```python
from build123d import *

# Parameters (mm, degrees)
SKETCH_1_R      = 2
SKETCH_1_R_2    = 1.5
SKETCH_1_R_3    = 5
SKETCH_1_R_4    = 0.95
SKETCH_1_W      = 8.2
SKETCH_1_H      = 4.2
EXTRUDE_1_DEPTH = 4


with BuildPart() as part:
    # 草图1 → 凸台-拉伸1 (new body)
    with BuildSketch(Plane.XY):
        with BuildLine():
            Line((-38.15, 66.25), (-38.15, 62.25))
            Line((-38.15, 62.25), (-39.45, 62.25))
            Line((-39.45, 62.25), (-39.45, 59.65))
            Line((-39.45, 59.65), (-38.15, 59.65))
            Line((-38.15, 59.65), (-38.15, 57.05))
            Line((-38.15, 57.05), (-35.15, 57.05))
            Line((-35.15, 57.05), (-35.15, 59.65))
            Line((-35.15, 59.65), (-33.85, 59.65))
            Line((-33.85, 59.65), (-33.85, 62.25))
            Line((-33.85, 62.25), (-35.15, 62.25))
            Line((-35.15, 62.25), (-35.15, 66.25))
            Line((-35.15, 66.25), (-25.65, 66.25))
            Line((-25.65, 66.25), (-25.65, 70.25))
            Line((-25.65, 70.25), (-17.65, 70.25))
            Line((-17.65, 70.25), (-17.65, 66.25))
            Line((-17.65, 66.25), (-8.15, 66.25))
            Line((-8.15, 66.25), (-8.15, 62.25))
            Line((-8.15, 62.25), (-9.45, 62.25))
            Line((-9.45, 62.25), (-9.45, 59.65))
            Line((-9.45, 59.65), (-8.15, 59.65))
            Line((-8.15, 59.65), (-8.15, 57.05))
            Line((-8.15, 57.05), (-5.15, 57.05))
            Line((-5.15, 57.05), (-5.15, 59.65))
            Line((-5.15, 59.65), (-3.85, 59.65))
            Line((-3.85, 59.65), (-3.85, 62.25))
            Line((-3.85, 62.25), (-5.15, 62.25))
            Line((-5.15, 62.25), (-5.15, 66.25))
            Line((-5.15, 66.25), (4.35, 66.25))
            Line((4.35, 66.25), (4.35, 57.55))
            Line((4.35, 57.55), (53.51460577, -41.768082641))
            ThreePointArc((53.51460577, -41.768082641), (38.475737517, -73.658373169), (10.85, -51.75))
            Line((10.85, -51.75), (-95.15, 57.55))
            Line((-95.15, 57.55), (-95.15, 66.25))
            Line((-95.15, 66.25), (-85.65, 66.25))
            Line((-85.65, 66.25), (-85.65, 70.25))
            Line((-85.65, 70.25), (-77.65, 70.25))
            Line((-77.65, 70.25), (-77.65, 66.25))
            Line((-77.65, 66.25), (-68.15, 66.25))
            Line((-68.15, 66.25), (-68.15, 62.25))
            Line((-68.15, 62.25), (-69.45, 62.25))
            Line((-69.45, 62.25), (-69.45, 59.65))
            Line((-69.45, 59.65), (-68.15, 59.65))
            Line((-68.15, 59.65), (-68.15, 57.05))
            Line((-68.15, 57.05), (-65.15, 57.05))
            Line((-65.15, 57.05), (-65.15, 59.65))
            Line((-65.15, 59.65), (-63.85, 59.65))
            Line((-63.85, 59.65), (-63.85, 62.25))
            Line((-63.85, 62.25), (-65.15, 62.25))
            Line((-65.15, 62.25), (-65.15, 66.25))
            Line((-65.15, 66.25), (-55.65, 66.25))
            Line((-55.65, 66.25), (-55.65, 70.25))
            Line((-55.65, 70.25), (-47.65, 70.25))
            Line((-47.65, 70.25), (-47.65, 66.25))
            Line((-47.65, 66.25), (-38.15, 66.25))
        make_face()
        with Locations((-20.262745434, 32.422010331)):
            Circle(SKETCH_1_R, mode=Mode.SUBTRACT)
        with Locations((6.598407643, -9.75)):
            Circle(SKETCH_1_R_2, mode=Mode.SUBTRACT)
        with Locations((33.35, -51.75)):
            Circle(SKETCH_1_R_3, mode=Mode.SUBTRACT)
        with Locations((33.35, -45.75)):
            Circle(SKETCH_1_R_4, mode=Mode.SUBTRACT)
        with Locations((33.35, -57.75)):
            Circle(SKETCH_1_R_4, mode=Mode.SUBTRACT)
        with Locations((-8.401592357, -9.75)):
            Rectangle(SKETCH_1_W, SKETCH_1_H, mode=Mode.SUBTRACT)
    extrude(amount=EXTRUDE_1_DEPTH)


solid = part.part
```
For this review, take the finished solid that the model builds, in its own axes (mm). A direction names the side the tool comes from. Round coordinates to 2 decimals unless told otherwise and drop trailing zeros. Write each loop counter-clockwise with the first axis right and the second up, starting at its lowest first coordinate (ties: lowest second). Pieces come first, ordered by that corner, then holes.
1) Take a section at C-C on x = -61. Give the boundary of the cut face in (y, z).
Answer below:
outline: (22.34, 0) - (66.25, 0) - (66.25, 4) - (22.34, 4) - close
2) For line 1 along X through (y, z) = (61, 1.45); line 2 along X through (y, z) = (-10.5, 1.4); line 3 along X through (y, z) = (33.5, 0.55), list the stretches that pass through material, from the lowest coordinate up.
Answer below:
line 1: x = -95.15 to -69.45, -63.85 to -39.45, -33.85 to -9.45, -3.85 to 4.35
line 2: x = -29.15 to -12.5, -4.3 to 5.3, 7.9 to 38.04
line 3: x = -71.83 to -21.95, -18.58 to 16.26
3) Mouldability with a two-part tool opening along Y and no side actions: class faces 4 (the face through (0, 66.25, 2)), 5 (the face through (-4.302, -10, 2)), 6 (the face through (4.35, 62, 2)), 7 (the face through (-18.415, 31.656, 1.972)) as +Y half, -Y half, draft (parallel to the pull), parting line (faces both ways), or undercut.
Answer below:
face 4: +Y half
face 5: undercut
face 6: draft
face 7: undercut
4) Take a section at A-A on z = 1.2. State how many separate pieces and enclosed holes the cut face has, then the cut area to 3 significant figures.
Answer below:
separate pieces: 1
enclosed holes: 6
area: 9,550 mm2
5) Machinability: for faces 1 (the face through (-47.65, 68, 2)), 2 (the face through (-90, 66.25, 2)), 3 (the face through (28.588, 8.586, 1.972)), which of the approach directions +Z, -Z, +X, -X, +Y, -Y give a long, thin tool a straight path to every point of the face, cutting with its end or side? Answer none if there is none.
Answer below:
face 1: +Z, -Z, +Y
face 2: +Z, -Z, -X, +Y
face 3: +Z, -Z, +X, +Y
6) Insertion check: pin 1 Ø1.3 at (y, z) = (58.5, 1.5) entering from +X; pin 2 Ø1.2 at (x, z) = (-12.5, 1.5) entering from +Y; pin 3 Ø1 at (x, z) = (-9, 1.5) entering from -Y; pin 4 Ø12 at (x, y) = (-2, -52.5) entering from -Z. Each pin has a flat end and moves straight along its axis. Give the tip position at first contact, or say it passes through.
Answer below:
pin 1: stops at x = 4.35
pin 2: stops at y = 66.25
pin 3: stops at y = -31.8
pin 4: passes through
7) Take a section at B-B on y = 18. Give the boundary of the cut face in (x, z), then the cut area to 3 significant figures.
Answer below:
outline: (-56.79, 0) - (23.93, 0) - (23.93, 4) - (-56.79, 4) - close
area: 323 mm2
